Here's how the part is built. I have some questions about the finished solid (model axes, mm). A direction names the side the tool comes from. Give positions to 0.01 mm unless a question says otherwise; leave off trailing zeros. Loops run counter-clockwise (first coordinate to the right, second up) from the corner with the lowest first, then second, coordinate; pieces in that order, holes last. Notation, with made-up numbers: (-26.5, 63.25) - (11.5, 63.25) arc R16 cw to (11.5, 67.25) - close; hole circle Ø7 at (-6, -16.75). An arc over 180 degrees is marked (long way). Return JSON: item names as keys, results as strings. Group by question number.
(1) I need wall thicknesses on probe 1 along Y at (x, z) = (-29.25, 29.3); probe 2 along Z at (x, y) = (-31, 6); probe 3 along Z at (x, y) = (15, 17). Which ranges of each line are inside material? Lowest first, please. Write a range as [from, to].
(2) If we section it at B-B (z = -28): Please give me the cut outline in (x, y).
(3) For P1, Ø1.1, axis at y = 17.5, z = 14.5, coming from the +X side; P2, Ø10, axis at x = -13.5, z = -15, coming from the -Y side; P3, Ø4, axis at y = 1, z = 13.5, coming from the -X side; P4, Ø2.5, axis at x = -29.25, y = 25, coming from the +Z side, each with a flat end and sliding along its axis, tell me the tip position at first contact or that it passes through.
(4) If we section it at C-C (x = 0): Please give me the cut outline in (y, z), then the cut area to 3 significant figures.
(5) If we section it at D-D (y = -7): Please give me the cut outline in (x, z).
(6) If we mould it in two halves opening along X, with no side actions, what happens to faces 1 (the cylindrical face through (18.5, -0.49, 6.05)), 2 (the flat face through (5, -1, -6)), 3 (the flat face through (20.9, -0.6, -5))? For each: released by +X, released by -X, zero draft, split by the parting line, or undercut.
(7) If we section it at A-A (y = -16): Please give me the cut outline in (x, z).
(8) On a 3-axis mill with a long thin cutter (end or side, diameter ignored), from which of +Z, -Z, +X, -X, +Y, -Y can I reach the whole of each face in a straight line? I mean faces 4 (the cylindrical face through (-25.5, -16, -8)), 5 (the flat face through (-21.6, -0.6, -5)), 6 (the cylindrical face through (0.1, -0.5, -22.5)), 7 (the flat face through (29, 16, 29)), 8 (the flat face through (-29, 16, 29)). Say none if no direction works.
```python
from build123d import *

# Parameters (mm, degrees)
SKETCH_1_W                       = 50
SKETCH_1_H                       = 1
SM_BASE_FLANGE_1_DEPTH           = 5
SM_EDGE_FLANGE_1_STRIP_W         = 9
SM_EDGE_FLANGE_1_STRIP_H         = 1
SM_EDGE_FLANGE_1_STRIP_CUT_DEPTH = 10
SM_EDGE_FLANGE_1_DEPTH           = 10
SM_BASE_FLANGE_1_2_DEPTH         = 1
SKETCH_12_W                      = 20
SKETCH_12_H                      = 30
SKETCH_12_W_2                    = 35
SKETCH_12_H_2                    = 10
SM_BASE_FLANGE_2_DEPTH           = 1
SM_EDGE_FLANGE_3_STRIP_W         = 9
SM_EDGE_FLANGE_3_STRIP_H         = 1
SM_EDGE_FLANGE_3_STRIP_CUT_DEPTH = 35
SM_EDGE_FLANGE_3_DEPTH           = 35
CUT_EXTRUDE_1_REACH              = 65.38
SKETCH_21_W                      = 25
SKETCH_21_H                      = 20
SM_EDGE_FLANGE_4_DEPTH           = 26.5
SM_EDGE_FLANGE_5_STRIP_W         = 9
SM_EDGE_FLANGE_5_STRIP_H         = 1
SM_EDGE_FLANGE_5_STRIP_CUT_DEPTH = 26.5
SM_EDGE_FLANGE_5_DEPTH           = 26.5
CUT_EXTRUDE_2_REACH              = 81.316
SKETCH_28_R                      = 1.5
FILLET_1_R                       = 3.5
CUT_EXTRUDE_3_REACH              = 59.879


# Sheet-metal steps are written as plain solids
with BuildPart() as part:
    # Sketch 1 → Sm Base Flange 1 (new, symmetric)
    with BuildSketch(Plane.XY):
        with Locations((0, -0.5)):
            Rectangle(SKETCH_1_W, SKETCH_1_H)
    extrude(amount=SM_BASE_FLANGE_1_DEPTH, both=True)

    # Sm Edge Flange 1 strip (across the edge) → Sm Edge Flange 1 strip cut (cut)
    with BuildSketch(Plane(origin=(-25, -1, 5), x_dir=(1, 0, 0), z_dir=(0, 0, -1))):
        with Locations((-2, -0.5)):
            Rectangle(SM_EDGE_FLANGE_1_STRIP_W, SM_EDGE_FLANGE_1_STRIP_H)
    sm_edge_flange_1_strip_cut = extrude(amount=SM_EDGE_FLANGE_1_STRIP_CUT_DEPTH, mode=Mode.SUBTRACT)

    # Sm Edge Flange 1 section (across the edge) → Sm Edge Flange 1 (add)
    with BuildSketch(Plane(origin=(-25, -1, 5), x_dir=(1, 0, 0), z_dir=(0, 0, -1))):
        with BuildLine():
            Line((-1, 2.5), (-1, 20))
            Line((-1, 20), (0, 20))
            Line((0, 20), (0, 2.5))
            ThreePointArc((0, 2.5), (0.732233047, 0.732233047), (2.5, 0))
            Line((2.5, 0), (2.5, -1))
            ThreePointArc((2.5, -1), (0.025126266, 0.025126266), (-1, 2.5))
        make_face()
    sm_edge_flange_1 = extrude(amount=SM_EDGE_FLANGE_1_DEPTH)

    # Sketch 9 → Sm Base Flange 1 2 (add)
    with BuildSketch(Plane.ZY.offset(26)):
        with BuildLine():
            Line((-5, -21), (-25, -21))
            ThreePointArc((-25, -21), (-30, -16), (-25, -11))
            Line((-25, -11), (-5, -11))
            Line((-5, -11), (-5, -21))
        make_face()
        with BuildLine():
            Line((-10, -18), (-25, -18))
            ThreePointArc((-25, -18), (-27, -16), (-25, -14))
            Line((-25, -14), (-10, -14))
            ThreePointArc((-10, -14), (-8, -16), (-10, -18))
        make_face(mode=Mode.SUBTRACT)
    sm_base_flange_1_2 = extrude(amount=-SM_BASE_FLANGE_1_2_DEPTH)

    # Mirror 1: Sm Edge Flange 1 strip cut, Sm Edge Flange 1, Sm Base Flange 1 2 across plane
    add(sm_edge_flange_1_strip_cut.mirror(Plane(origin=(0, 0, 0), x_dir=(0, 0, 1), z_dir=(1, 0, 0))), mode=Mode.SUBTRACT)
    add(sm_edge_flange_1.mirror(Plane(origin=(0, 0, 0), x_dir=(0, 0, 1), z_dir=(1, 0, 0))))
    add(sm_base_flange_1_2.mirror(Plane(origin=(0, 0, 0), x_dir=(0, 0, 1), z_dir=(1, 0, 0))))

    # Sketch 12 → Sm Base Flange 2 (add)
    with BuildSketch(Plane.XZ.offset(1)):
        with Locations((0, -20)):
            Rectangle(SKETCH_12_W, SKETCH_12_H)
        with Locations((0, 10)):
            Rectangle(SKETCH_12_W_2, SKETCH_12_H_2)
    extrude(amount=-SM_BASE_FLANGE_2_DEPTH)

    # Sm Edge Flange 3 strip (across the edge) → Sm Edge Flange 3 strip cut (cut)
    with BuildSketch(Plane(origin=(-17.5, 0, 15), x_dir=(0, 0, -1), z_dir=(1, 0, 0))):
        with Locations((-1, -0.5)):
            Rectangle(SM_EDGE_FLANGE_3_STRIP_W, SM_EDGE_FLANGE_3_STRIP_H)
    extrude(amount=SM_EDGE_FLANGE_3_STRIP_CUT_DEPTH, mode=Mode.SUBTRACT)

    # Sm Edge Flange 3 section (across the edge) → Sm Edge Flange 3 (add)
    with BuildSketch(Plane(origin=(-17.5, 0, 15), x_dir=(0, 0, -1), z_dir=(1, 0, 0))):
        with BuildLine():
            Line((0, 2.5), (0, 29))
            Line((0, 29), (1, 29))
            Line((1, 29), (1, 2.5))
            ThreePointArc((1, 2.5), (1.732233047, 0.732233047), (3.5, 0))
            Line((3.5, 0), (3.5, -1))
            ThreePointArc((3.5, -1), (1.025126266, 0.025126266), (0, 2.5))
        make_face()
    extrude(amount=SM_EDGE_FLANGE_3_DEPTH)

    # Sketch 21 → Cut-Extrude 1 (cut, up to next)
    with BuildSketch(Plane.XY.offset(15), mode=Mode.PRIVATE) as cut_extrude_1_sk1:
        with Locations((0, 19)):
            Rectangle(SKETCH_21_W, SKETCH_21_H)
    cut_extrude_1_tool1 = extrude(cut_extrude_1_sk1.sketch, amount=-CUT_EXTRUDE_1_REACH, mode=Mode.PRIVATE) & part.part
    add(cut_extrude_1_tool1.solids().sort_by_distance((0, 19, 15))[0], mode=Mode.SUBTRACT)

    # Sm Edge Flange 4 section (across the edge) → Sm Edge Flange 4 (add)
    with BuildSketch(Plane(origin=(-20, 29, 15), x_dir=(1, 0, 0), z_dir=(0, -1, 0))):
        with BuildLine():
            Line((-1, 2.5), (-1, 14))
            Line((-1, 14), (0, 14))
            Line((0, 14), (0, 2.5))
            ThreePointArc((0, 2.5), (0.732233047, 0.732233047), (2.5, 0))
            Line((2.5, 0), (2.5, -1))
            ThreePointArc((2.5, -1), (0.025126266, 0.025126266), (-1, 2.5))
        make_face()
    sm_edge_flange_4 = extrude(amount=SM_EDGE_FLANGE_4_DEPTH)

    # Sm Edge Flange 5 strip (across the edge) → Sm Edge Flange 5 strip cut (cut)
    with BuildSketch(Plane(origin=(-21, 2.5, 29), x_dir=(0, 0, -1), z_dir=(0, 1, 0))):
        with Locations((-2, -0.5)):
            Rectangle(SM_EDGE_FLANGE_5_STRIP_W, SM_EDGE_FLANGE_5_STRIP_H)
    sm_edge_flange_5_strip_cut = extrude(amount=SM_EDGE_FLANGE_5_STRIP_CUT_DEPTH, mode=Mode.SUBTRACT)

    # Sm Edge Flange 5 section (across the edge) → Sm Edge Flange 5 (add)
    with BuildSketch(Plane(origin=(-21, 2.5, 29), x_dir=(0, 0, -1), z_dir=(0, 1, 0))):
        with BuildLine():
            Line((-1, 2.5), (-1, 14))
            Line((-1, 14), (0, 14))
            Line((0, 14), (0, 2.5))
            ThreePointArc((0, 2.5), (0.732233047, 0.732233047), (2.5, 0))
            Line((2.5, 0), (2.5, -1))
            ThreePointArc((2.5, -1), (0.025126266, 0.025126266), (-1, 2.5))
        make_face()
    sm_edge_flange_5 = extrude(amount=SM_EDGE_FLANGE_5_DEPTH)

    # Sketch 28 → Cut-Extrude 2 (cut, up to next)
    with BuildSketch(Plane.XY.offset(30), mode=Mode.PRIVATE) as cut_extrude_2_sk1:
        with Locations((-29.25, 25)):
            Circle(SKETCH_28_R)
    cut_extrude_2_tool1 = extrude(cut_extrude_2_sk1.sketch, amount=-CUT_EXTRUDE_2_REACH, mode=Mode.PRIVATE) & part.part
    # Sketch 28 → Cut-Extrude 2 (cut, up to next)
    with BuildSketch(Plane.XY.offset(30), mode=Mode.PRIVATE) as cut_extrude_2_sk2:
        with Locations(Location((-29.25, 6.5, 0), (0, 0, 180))):
            Circle(SKETCH_28_R)
    cut_extrude_2_tool2 = extrude(cut_extrude_2_sk2.sketch, amount=-CUT_EXTRUDE_2_REACH, mode=Mode.PRIVATE) & part.part
    cut_extrude_2_1 = cut_extrude_2_tool1.solids().sort_by_distance((-29.25, 25, 30))[0]
    add(cut_extrude_2_1, mode=Mode.SUBTRACT)
    cut_extrude_2_2 = cut_extrude_2_tool2.solids().sort_by_distance((-29.25, 6.5, 30))[0]
    add(cut_extrude_2_2, mode=Mode.SUBTRACT)
    cut_extrude_2 = cut_extrude_2_1 + cut_extrude_2_2  # Cut-Extrude 2 as one shape, for the pattern or mirror that repeats it

    # Mirror 2: Sm Edge Flange 4, Sm Edge Flange 5 strip cut, Sm Edge Flange 5, Cut-Extrude 2 across plane
    add(sm_edge_flange_4.mirror(Plane(origin=(0, 0, 0), x_dir=(0, 0, 1), z_dir=(1, 0, 0))))
    add(sm_edge_flange_5_strip_cut.mirror(Plane(origin=(0, 0, 0), x_dir=(0, 0, 1), z_dir=(1, 0, 0))), mode=Mode.SUBTRACT)
    add(sm_edge_flange_5.mirror(Plane(origin=(0, 0, 0), x_dir=(0, 0, 1), z_dir=(1, 0, 0))))
    add(cut_extrude_2.mirror(Plane(origin=(0, 0, 0), x_dir=(0, 0, 1), z_dir=(1, 0, 0))), mode=Mode.SUBTRACT)

    # Fillet 1
    fillet_1_edges = [part.edges().sort_by_distance(p)[0] for p in [
        (17.5, -0.5, 5),
        (-17.5, -0.5, 5),
        (12.5, 29, 14.5),
        (12.5, 9, 14.5),
        (-12.5, 9, 14.5),
        (-12.5, 29, 14.5),
        (-35, 2.5, 29.5),
        (-35, 29, 29.5),
        (35, 29, 29.5),
        (35, 2.5, 29.5),
        (-25.5, -21, 5),
        (25.5, -21, 5),
    ]]
    fillet(fillet_1_edges, radius=FILLET_1_R)

    # Sketch 29 → Cut-Extrude 3 (cut, up to next)
    with BuildSketch(Plane.XZ.offset(1), mode=Mode.PRIVATE) as cut_extrude_3_sk1:
        with BuildLine():
            Line((2.5, 0), (2.5, -20))
            ThreePointArc((2.5, -20), (0, -22.5), (-2.5, -20))
            Line((-2.5, -20), (-2.5, 0))
            ThreePointArc((-2.5, 0), (0, 2.5), (2.5, 0))
        make_face()
    cut_extrude_3_tool1 = extrude(cut_extrude_3_sk1.sketch, amount=-CUT_EXTRUDE_3_REACH, mode=Mode.PRIVATE) & part.part
    add(cut_extrude_3_tool1.solids().sort_by_distance((0, -1, -10))[0], mode=Mode.SUBTRACT)


solid = part.part
```
Values:
{
 "1": {"probe 1": "[2.5, 5], [8, 23.5], [26.5, 29]", "probe 2": "[29, 30]", "probe 3": "[14, 15]"},
 "2": {"outline": "(-26, -20) - (-25, -20) - (-25, -12) - (-26, -12) - close; (-10, -1) - (10, -1) - (10, 0) - (-10, 0) - close; (25, -20) - (26, -20) - (26, -12) - (25, -12) - close"},
 "3": {"P1": "x = 20", "P2": "y = -1", "P3": "x = -19.75", "P4": "through"},
 "4": {"outline": "(-1, -35) - (0, -35) - (0, -22.5) - (-1, -22.5) - close; (-1, 2.5) - (0, 2.5) - (0, 11.5) arc R2.5 cw to (2.5, 14) - (9, 14) - (9, 15) - (2.5, 15) arc R3.5 ccw to (-1, 11.5) - close", "area": "32.7 mm2"},
 "5": {"outline": "(-26, -5) - (-25, -5) - (-25, 5) - (-26, 5) - close; (25, -5) - (26, -5) - (26, 5) - (25, 5) - close"},
 "6": {"face 1": "released by +X", "face 2": "undercut", "face 3": "zero draft"},
 "7": {"outline": "(-26, -30) - (-25, -30) - (-25, -27) - (-26, -27) - close; (-26, -8) - (-25, -8) - (-25, 5) - (-26, 5) - close; (25, -30) - (26, -30) - (26, -27) - (25, -27) - close; (25, -8) - (26, -8) - (26, 5) - (25, 5) - close"},
 "8": {"face 4": "+X, -X", "face 5": "-Z, -X, +Y", "face 6": "+Y, -Y", "face 7": "-Z, +X, +Y, -Y", "face 8": "-Z, -X, +Y, -Y"}
}
